Source: CAD feature listing. Evaluate the final solid. Frame: model axes, mm. Round coordinates to 2 decimals unless told otherwise and drop trailing zeros. Write each loop counter-clockwise with the first axis right and the second up, starting at its lowest first coordinate (ties: lowest second). Pieces come first, ordered by that corner, then holes. Notation, with made-up numbers: M 74,34.5 L 131,34.5 A22 ccw 131,63.5 Z; hole C -40,28 d9. An arc over 180 degrees is marked long. Answer in a Markdown table with one row per item. Add a question column.
Item 1: Cut plane B-B on y = 1.8. Give the number of separate pieces and of enclosed holes in the cut face, and give its area (3 significant figures).
Item 2: Cut plane A-A on x = 44.5. Return loops of the section in (y, z) (3 decimals).
Item 3: Material intervals for probe 1 along X at (y, z) = (1.75, -40.5) (3 decimals); probe 2 along Z at (x, y) = (20, 2.4); probe 3 along Z at (x, y) = (29, 0.8) (3 decimals), sorted ascending.
Item 4: Contact query for flat-ended pins moving along their axis: pin 1 (1.6 mm diameter, centred on y = 1, z = -14, fed in from +X); pin 2 (1.6 mm diameter, centred on x = 20.5, y = 1, fed in from -Z); pin 3 (1.6 mm diameter, centred on y = 1.5, z = -44, fed in from +X). Output: stop coordinate, or through.
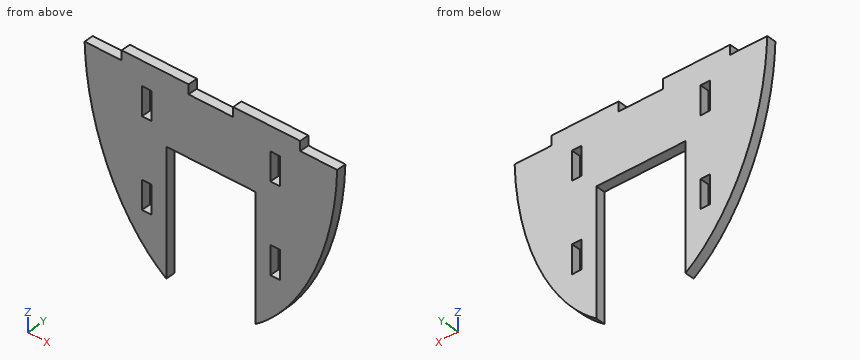
from build123d import *

# Parameters (mm, degrees)
BOSS_EXTRUDE1_DEPTH = 3.175
SKETCH2_W           = 3.175
SKETCH2_H           = 9.492
SKETCH2_W_2         = 12.5
SKETCH2_H_2         = 3.175
SKETCH2_W_3         = 15
SKETCH2_W_4         = 30
SKETCH2_H_3         = 55.059917187
CUT_EXTRUDE1_DEPTH  = 4.1750001


with BuildPart() as part:
    # Sketch1 → Boss-Extrude1 (new body)
    with BuildSketch(Plane(origin=(0, 0, 0), x_dir=(1, 0, 0), z_dir=(0, 1, 0))):
        with BuildLine():
            add(Edge.make_bspline(
                [(0, 0), (0, 36), (20.5, 67.166666667), (40.5, 70), (42.5, 70)],
                knots=[0, 0, 0, 0, 0.45, 0.5, 0.5, 0.5, 0.5], degree=3))
            Line((0, 0), (42.5, 0))
            Line((42.5, 0), (42.5, 70))
        make_face()
        with BuildLine():
            Line((42.5, 70), (42.5, 0))
            Line((42.5, 0), (85, 0))
            add(Edge.make_bspline(
                [(42.5, 70), (44.5, 70), (64.5, 67.166666667), (85, 36), (85, 0)],
                knots=[0.5, 0.5, 0.5, 0.5, 0.55, 1, 1, 1, 1], degree=3))
        make_face()
    extrude(amount=BOSS_EXTRUDE1_DEPTH)

    # Sketch2 → Cut-Extrude1 (cut, through all)
    with BuildSketch(Plane(origin=(0, 3.175, 0), x_dir=(1, 0, 0), z_dir=(0, 1, 0))):
        with Locations((20.9125, 42.246)):
            Rectangle(SKETCH2_W, SKETCH2_H)
        with Locations((64.0875, 42.246)):
            Rectangle(SKETCH2_W, SKETCH2_H)
        with Locations((20.9125, 12.754)):
            Rectangle(SKETCH2_W, SKETCH2_H)
        with Locations((64.0875, 12.754)):
            Rectangle(SKETCH2_W, SKETCH2_H)
        with Locations((6.25, 1.5875)):
            Rectangle(SKETCH2_W_2, SKETCH2_H_2)
        with Locations((42.5, 1.5875)):
            Rectangle(SKETCH2_W_3, SKETCH2_H_2)
        with Locations((78.75, 1.5875)):
            Rectangle(SKETCH2_W_2, SKETCH2_H_2)
        with Locations((42.5, 50.704958594)):
            Rectangle(SKETCH2_W_4, SKETCH2_H_3)
    extrude(amount=-CUT_EXTRUDE1_DEPTH, mode=Mode.SUBTRACT)


solid = part.part
Results below:
| question | item | result |
|---|---|---|
| 1 | separate pieces | 1 |
| 1 | enclosed holes | 4 |
| 1 | area | 2,990 mm2 |
| 2 | outline | M 0,-23.175 L 3.175,-23.175 L 3.175,-3.175 L 0,-3.175 Z |
| 3 | probe 1 | 8.578 to 19.325, 22.5 to 27.5, 57.5 to 62.5, 65.675 to 76.422 |
| 3 | probe 2 | -58.07 to -46.99, -37.5 to -17.5, -8.01 to 0 |
| 3 | probe 3 | -23.175 to 0 |
| 4 | pin 1 | x = 84.16 |
| 4 | pin 2 | z = -59.44 |
| 4 | pin 3 | x = 75.11 |
